```python
from build123d import *

# Parameters (mm, degrees)
F1_DEPTH = 8.128
F2_W     = 29.380368
F2_H     = 8.890002
F3_DEPTH = 25.4
F4_W     = 6.938537
F4_H     = 17.482635
F5_DEPTH = 8.382
F6_W     = 8.456341
F6_H     = 17.265804
F7_DEPTH = 9.906


with BuildPart() as f1:
    # F0 (on Front) → F1 (new body)
    with BuildSketch(Plane.XZ):
        Polygon((0, 5.420732), (0, 0), (0, -22.550246), (29.380368, -22.550246), (29.380368, 4.987073), (23.525976, 4.987073), (23.525976, 0), (6.396465, 0), (6.396465, 5.420732), align=None)
    extrude(amount=F1_DEPTH)

    # F2 (on face) → F3 (join)
    with BuildSketch(Plane.XZ.offset(8.128)):
        with Locations((14.690184, -18.105245)):
            Rectangle(F2_W, F2_H)
    extrude(amount=F3_DEPTH)

    # F4 (on face) → F5 (join)
    with BuildSketch(Plane.XY.offset(-13.660244)):
        with Locations((15.286463, -24.786682)):
            Rectangle(F4_W, F4_H)
    extrude(amount=-F5_DEPTH)

    # F6 (on face) → F7 (cut)
    with BuildSketch(Plane.XY.offset(-13.660244)):
        with Locations((14.527561, -24.895098)):
            Rectangle(F6_W, F6_H)
    extrude(amount=-F7_DEPTH, mode=Mode.SUBTRACT)


solid = f1.part
```
For this review, take the finished solid that the model builds, in its own axes (mm). A direction names the side the tool comes from. Coordinates: 2 decimals unless noted, no trailing zeros. Order: outer loops, then holes, each group sorted by start corner. A loop starts at its lowest first (then second) coordinate and runs counter-clockwise, first axis right, second up. Notation, with made-up numbers: (77.25, -14) - (129.25, -14) arc R31 ccw to (129.25, 15) - close; hole circle Ø7 at (-26, -15). An arc over 180 degrees is marked (long way). Answer as a JSON object with one key per item and string values. Group by question number.
1. We need section B-B on z = -14.25. State the section outline as (x, y) points, then the cut area to 3 significant figures.
2. Clearance check with flat-ended pins moving along their axes: P1, Ø4, axis at x = 11, y = -5.5, coming from the +Z side; P2, Ø4.5, axis at x = 26.5, y = -5.5, coming from the +Z side; P3, Ø6, axis at x = 15, y = -15.5, coming from the +Z side. State where each tip first meets the part, or that it passes through.
3. We need section D-D on x = 13.5. State the section outline as (y, z) points, then the cut area to 3 significant figures.
4. For probe 1 along Y at (x, z) = (7.75, -1.75); probe 2 along X at (y, z) = (-2, 2); probe 3 along Y at (x, z) = (16.5, -13.75), list the stretches that pass through material, from the lowest coordinate up.
5. We need section C-C on z = 3.5. State the section outline as (x, y) points, then the cut area to 3 significant figures.
6. The part is to be moulded in two halves that separate along X. For faces 1 (the flat face through (0, -13, -15)), 2 (the flat face through (14, -16.262, -18)), 3 (the flat face through (14, 0, -8)), say which applies: pulls with the +X half, pulls with the -X half, needs draft (parallel to the pull), parting line crosses it, or undercut.
7. We need section A-A on y = -18. State the section outline as (x, z) points.
8. For faces 4 (the flat face through (14, -15, -13.66)), 5 (the flat face through (26, -4, 4.987)), 6 (the flat face through (10.299, -25, -18)), list the 3-axis set-ups (+Z, -Z, +X, -X, +Y, -Y) from which the entire face can be reached by the end or side of a thin tool; tool diameter is ignored.
Final values:
{
 "1": {"outline": "(0, -33.53) - (10.3, -33.53) - (10.3, -16.26) - (18.76, -16.26) - (18.76, -33.53) - (29.38, -33.53) - (29.38, 0) - (0, 0) - close", "area": "839 mm²"},
 "2": {"P1": "z = 0", "P2": "z = 4.99", "P3": "z = -13.66"},
 "3": {"outline": "(-16.26, -22.55) - (0, -22.55) - (0, 0) - (-8.13, 0) - (-8.13, -13.66) - (-16.26, -13.66) - close", "area": "256 mm²"},
 "4": {"probe 1": "-8.13 to 0", "probe 2": "0 to 6.4, 23.53 to 29.38", "probe 3": "-16.26 to 0"},
 "5": {"outline": "(0, -8.13) - (6.4, -8.13) - (6.4, 0) - (0, 0) - close; (23.53, -8.13) - (29.38, -8.13) - (29.38, 0) - (23.53, 0) - close", "area": "99.6 mm²"},
 "6": {"face 1": "pulls with the -X half", "face 2": "undercut", "face 3": "needs draft"},
 "7": {"outline": "(0, -22.55) - (10.3, -22.55) - (10.3, -13.66) - (0, -13.66) - close; (18.76, -22.55) - (29.38, -22.55) - (29.38, -13.66) - (18.76, -13.66) - close"},
 "8": {"face 4": "+Z, +X, -X, -Y", "face 5": "+Z, +X, +Y, -Y", "face 6": "+Z, -Z, -Y"}
}
